Part model, mm, in its own coordinate system. Face numbers are marked on the shaded views. A direction names the side the tool comes from. Round coordinates to 2 decimals unless told otherwise and drop trailing zeros. Write each loop counter-clockwise with the first axis right and the second up, starting at its lowest first coordinate (ties: lowest second). Pieces come first, ordered by that corner, then holes. Notation, with made-up numbers: M 27.5,-11 L 54.5,-11 A22 ccw 54.5,12 Z; hole C -2.5,-18.75 d5. An arc over 180 degrees is marked long. Use one line per item in the form item = value. Start each with the question number.
Item 1: Flat gauge pin, fed straight in: pin 1 Ø1.4 at (x, z) = (24, -1) entering from -Y. Where does the tip first touch, or does it go through?
Item 2: Probe L1, parallel to X at y = 0.8, z = -4.5; L2, parallel to Z at x = 21, y = 1.85; L3, parallel to Z at x = 18, y = 0.1. List the from-to ranges inside material, lowest first.
Item 3: Cut at B-B, the plane z = 6.25. Give the cut face in (x, y), then the cut area to 3 significant figures.
Item 4: Which spindle directions (+Z, -Z, +X, -X, +Y, -Y) get a long thin tool onto all of the face, cutting with end or side? Do the marked faces 5 and 6. Say none if no direction does.
Item 5: Cut at D-D, the plane x = 28.5. Give the cut face in (y, z).
Item 6: Cut at A-A, the plane y = 1.35. Give the cut face in (x, z).
Item 7: Cut at C-C, the plane x = 15.5. Give the cut face in (y, z), then the cut area to 3 significant figures.
Item 8: Mould opens along X. For the marked faces 1, 2, 3 and 4 say: +X half, -X half, draft (parallel to the pull), parting line (faces both ways), or undercut.
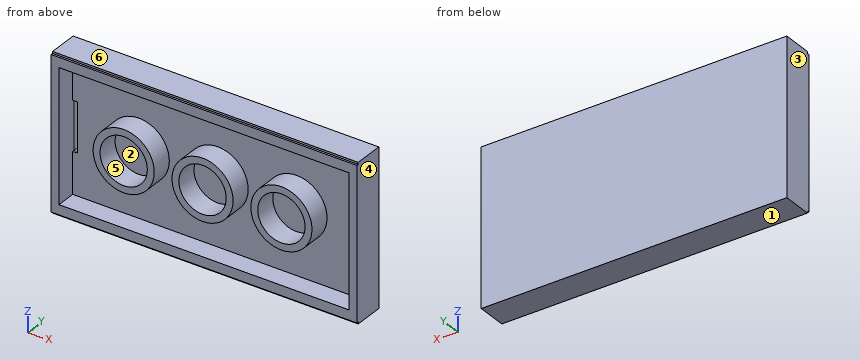
from build123d import *

# Parameters (mm, degrees)
MAINBASESKETCH_W              = 47.8
MAINBASESKETCH_H              = 3.2
MAINBASEEXTRUDE_DEPTH         = 7.9
MAINBASESHELL_T               = -1.2
UNDERSIDECIRCLEEXT_START      = -0.2
UNDERSIDECIRCLESKETCH_R       = 3.1
UNDERSIDECIRCLESKETCH_R_2     = 2.4
UNDERSIDECIRCLEEXT_DEPTH      = 2.4
UNDERSIDECIRCLEPATTERN_COUNT  = 3
UNDERSIDECIRCLEPATTERN_PITCH  = 8
EXTENDEDBASEEDGECUT_DEPTH     = 0.2
EXTENDEDBASEEDGECUT2_DEPTH    = 0.2
EXTENDEDBASEEDGECUT3_DEPTH    = 0.2
EXTENDEDBASEEDGESKETCH4_W     = 47.4
EXTENDEDBASEEDGESKETCH4_H     = 0.199766916
EXTENDEDBASEEDGECUT4_DEPTH    = 0.2
EXTENDEDNBASEUNDERNOTCH_DEPTH = 0.4
EXTENDEBASENOTCHFILLET_R      = 0.2
CUT_EXTRUDE60_DEPTH           = 50.170632952
CUT_EXTRUDE60_DEPTH_BACK      = 50.170632952
SKETCH178_W                   = 15.972643613
SKETCH178_H                   = 15.8
SKETCH179_W                   = 1.2
SKETCH179_H                   = 13.4
SKETCH180_W                   = 0.411945133
SKETCH180_H                   = 15.8
CUT_EXTRUDE61_DEPTH           = 34.627758191


with BuildPart() as part:
    # MainBaseSketch → MainBaseExtrude (new, symmetric)
    with BuildSketch(Plane.XY):
        with Locations((24.581967213, 1.6)):
            Rectangle(MAINBASESKETCH_W, MAINBASESKETCH_H)
    extrude(amount=MAINBASEEXTRUDE_DEPTH, both=True)

    # MainBaseShell
    mainbaseshell_openings = [part.faces().sort_by_distance(p)[0] for p in [
        (24.581967213, 0, 0),
    ]]
    offset(amount=MAINBASESHELL_T, openings=mainbaseshell_openings, kind=Kind.INTERSECTION)

    # UnderSideCircleSketch → UnderSideCircleExt (add)
    with BuildSketch(Plane.XZ.offset(-2).offset(UNDERSIDECIRCLEEXT_START)):
        with Locations((8.581967213, 0)):
            Circle(UNDERSIDECIRCLESKETCH_R)
        with Locations((8.581967213, 0)):
            Circle(UNDERSIDECIRCLESKETCH_R_2, mode=Mode.SUBTRACT)
    undersidecircleext = extrude(amount=UNDERSIDECIRCLEEXT_DEPTH)

    # UnderSideCirclePattern: UnderSideCircleExt ×3
    with Locations(*[(i * UNDERSIDECIRCLEPATTERN_PITCH, 0, 0) for i in range(1, UNDERSIDECIRCLEPATTERN_COUNT)]):
        add(undersidecircleext)

    # ExtendedBaseEdgeSketch → ExtendedBaseEdgeCut (cut)
    with BuildSketch(Plane.ZY.offset(-0.681967213)):
        Polygon((-7.9, 0), (-7.9, 0.199766916), (-7.702184024, 0.199766916), (7.702184024, 0.199766916), (7.9, 0.199766916), (7.9, 0), (7.702184024, 0), (-7.702184024, 0), align=None)
    extrude(amount=-EXTENDEDBASEEDGECUT_DEPTH, mode=Mode.SUBTRACT)

    # ExtendedBaseEdgeSketch2 → ExtendedBaseEdgeCut2 (cut)
    with BuildSketch(Plane(origin=(0, 0, -7.9), x_dir=(-1, 0, 0), z_dir=(0, 0, -1))):
        Polygon((-48.481967213, 0), (-48.481967213, 0.203418418), (-0.881967213, 0.199766916), (-0.881967213, 0), align=None)
    extrude(amount=-EXTENDEDBASEEDGECUT2_DEPTH, mode=Mode.SUBTRACT)

    # ExtendedBaseEdgeSketch3 → ExtendedBaseEdgeCut3 (cut)
    with BuildSketch(Plane(origin=(48.481967213, 0, 0), x_dir=(0, 0, -1), z_dir=(1, 0, 0))):
        Polygon((-7.9, 0), (-7.9, 0.199766916), (7.7, 0.203418418), (7.7, 0), align=None)
    extrude(amount=-EXTENDEDBASEEDGECUT3_DEPTH, mode=Mode.SUBTRACT)

    # ExtendedBaseEdgeSketch4 → ExtendedBaseEdgeCut4 (cut)
    with BuildSketch(Plane.XY.offset(7.9)):
        with Locations((24.581967213, 0.099883458)):
            Rectangle(EXTENDEDBASEEDGESKETCH4_W, EXTENDEDBASEEDGESKETCH4_H)
    extrude(amount=-EXTENDEDBASEEDGECUT4_DEPTH, mode=Mode.SUBTRACT)

    # ExtendedbaseUnderNotchSketch → ExtendednbaseUnderNotch (cut)
    with BuildSketch(Plane.XZ.offset(-2)):
        Polygon((1.881967213, 0), (1.881967213, 2.502100162), (2.381942481, 2.502100162), (2.381942481, -2.499482153), (1.881967213, -2.499482153), align=None)
    extrude(amount=-EXTENDEDNBASEUNDERNOTCH_DEPTH, mode=Mode.SUBTRACT)

    # ExtendebaseNotchFillet
    extendebasenotchfillet_edges = [part.edges().sort_by_distance(p)[0] for p in [
        (1.881967213, 2.4, 0.001309004),
        (2.131954847, 2.4, 2.502100162),
        (2.381942481, 2.4, 0.001309004),
        (2.131954847, 2.4, -2.499482153),
    ]]
    fillet(extendebasenotchfillet_edges, radius=EXTENDEBASENOTCHFILLET_R)

    # Sketch178 → Cut-Extrude60 (cut, two sides: drawn at the far end of the back side and taken through both)
    with BuildSketch(Plane(origin=(0, 2, 0), x_dir=(-1, 0, 0), z_dir=(0, -1, 0)).offset(-CUT_EXTRUDE60_DEPTH_BACK)):
        with Locations((-40.495645407, 0)):
            Rectangle(SKETCH178_W, SKETCH178_H)
    extrude(amount=CUT_EXTRUDE60_DEPTH + CUT_EXTRUDE60_DEPTH_BACK, mode=Mode.SUBTRACT)

    # Sweep29: sweep along a curve in space
    with BuildLine() as sweep29_path:
        Line((32.5093236, 0, 6.7), (32.5093236, 2, 6.7))
    # Sketch179 → Sweep29 (sweep)
    with BuildSketch(Plane.XZ):
        with Locations((31.9093236, 0)):
            Rectangle(SKETCH179_W, SKETCH179_H)
    sweep(path=sweep29_path.line)

    # Sketch180 → Cut-Extrude61 (cut, through all)
    with BuildSketch(Plane(origin=(0, 3.2, 0), x_dir=(1, 0, 0), z_dir=(0, 1, 0))):
        with Locations((0.88793978, 0)):
            Rectangle(SKETCH180_W, SKETCH180_H)
        with Locations((32.303351034, 0)):
            Rectangle(SKETCH180_W, SKETCH180_H)
    extrude(amount=-CUT_EXTRUDE61_DEPTH, mode=Mode.SUBTRACT)


solid = part.part
Model answer:
q1.pin_1 = 2
q2.L1 = 1.09 to 1.88, 31.31 to 32.1
q2.L2 = -7.9 to -6.7, 6.7 to 7.9
q2.L3 = -7.7 to -6.7, -2.76 to -1.94, 1.94 to 2.76, 6.7 to 7.7
q3.outline = M 1.09,0 L 1.88,0 L 1.88,2 L 31.31,2 L 31.31,0 L 32.1,0 L 32.1,3.2 L 1.09,3.2 Z
q3.area = 40.4 mm²
q4.face_5 = -Y
q4.face_6 = +Z, +X, -X, +Y, -Y
q5.outline = M 0,-7.7 L 0.2,-7.7 L 0.2,-7.9 L 3.2,-7.9 L 3.2,7.9 L 0.2,7.9 L 0.2,7.7 L 0,7.7 L 0,6.7 L 2,6.7 L 2,-6.7 L 0,-6.7 Z
q6.outline = M 1.09,-7.9 L 32.1,-7.9 L 32.1,7.9 L 1.09,7.9 Z; C 8.58,0 d6.2; C 16.58,0 d6.2; C 24.58,0 d6.2; hole M 1.88,-6.7 L 31.31,-6.7 L 31.31,6.7 L 1.88,6.7 Z; hole C 8.58,0 d4.8; hole C 16.58,0 d4.8; hole C 24.58,0 d4.8
q7.outline = M -0.2,-2.91 L 2,-2.91 L 2,-6.7 L 0,-6.7 L 0,-7.7 L 0.2,-7.7 L 0.2,-7.9 L 3.2,-7.9 L 3.2,7.9 L 0.2,7.9 L 0.2,7.7 L 0,7.7 L 0,6.7 L 2,6.7 L 2,2.91 L -0.2,2.91 L -0.2,2.14 L 2,2.14 L 2,-2.14 L -0.2,-2.14 Z
q7.area = 27.0 mm²
q8.face_1 = draft
q8.face_2 = undercut
q8.face_3 = -X half
q8.face_4 = +X half
